Read the model definition and answer for the solid it produces. Units are mm, in the model's axes. Face numbers are marked on the shaded views. A direction names the side the tool comes from. Coordinates: 2 decimals unless noted, no trailing zeros. Loops run counter-clockwise (first coordinate to the right, second up) from the corner with the lowest first, then second, coordinate; pieces in that order, holes last.
Q1. Section C-C (y = 2.25) is taken. Give the vertices of the cut face in (x, z).
Q2. Flat-ended cylindrical pins translate along their axes: P1, Ø1.5, axis at y = 2.5, z = -3.5, coming from the +X side; P2, Ø3, axis at y = 8.5, z = 10, coming from the -X side; P3, Ø8, axis at x = -60.5, z = -10, coming from the -Y side. Find the tip coordinate at first contact, or state that the pin passes through.
Q3. Section D-D (z = -10.5) is taken. Give the vertices of the cut face in (x, y), then the cut area to 3 significant figures.
Q4. Section A-A (z = 0) is taken. Give the vertices of the cut face in (x, y), then the cut area to 3 significant figures.
Q5. Straight lines are drawn through the part: line 1 (Z direction, x = 5, y = 21.25); line 2 (X direction, y = 3.75, z = -0.25); line 3 (Z direction, x = 8, y = 21.75). For each, find the intervals that lie inside material, in ascending order.
Q6. Section B-B (y = 11.3) is taken. Give the vertices of the cut face in (x, z), then the cut area to 3 significant figures.
Q7. Which of the six approach directions +Z, -Z, +X, -X, +Y, -Y give full straight-line access (tool end or side, diameter ignored) to the marked faces 1 and 2?
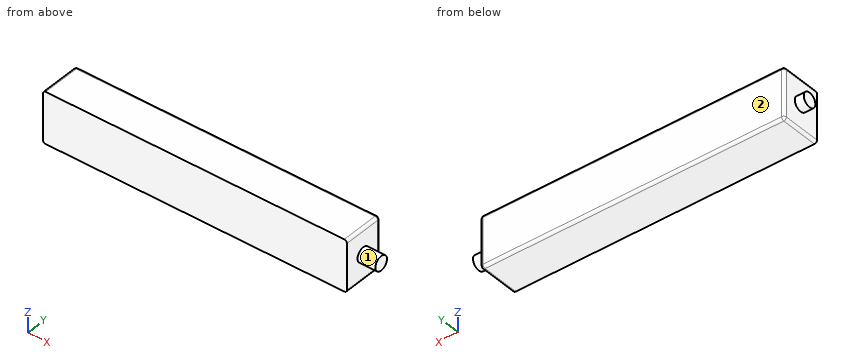
from build123d import *

# Parameters (mm, degrees)
SKETCH1_W           = 170
SKETCH1_H           = 28.6
BOSS_EXTRUDE1_DEPTH = 22.6
SKETCH2_R           = 4
BOSS_EXTRUDE2_DEPTH = 10
SKETCH3_R           = 4
BOSS_EXTRUDE3_DEPTH = 5
FILLET1_R           = 1.5


with BuildPart() as part:
    # Sketch1 → Boss-Extrude1 (new body)
    with BuildSketch(Plane(origin=(0, 0, 0), x_dir=(1, 0, 0), z_dir=(0, 1, 0))):
        Rectangle(SKETCH1_W, SKETCH1_H)
    extrude(amount=BOSS_EXTRUDE1_DEPTH)

    # Sketch2 → Boss-Extrude2 (add)
    with BuildSketch(Plane(origin=(85, 0, 0), x_dir=(0, 0, -1), z_dir=(1, 0, 0))):
        with Locations((0, 11.3)):
            Circle(SKETCH2_R)
    extrude(amount=BOSS_EXTRUDE2_DEPTH)

    # Sketch3 → Boss-Extrude3 (add)
    with BuildSketch(Plane.ZY.offset(85)):
        with Locations((0, 11.3)):
            Circle(SKETCH3_R)
    extrude(amount=BOSS_EXTRUDE3_DEPTH)

    # Fillet1
    fillet1_edges = [part.edges().sort_by_distance(p)[0] for p in [
        (85, 22.6, 0),
        (0, 22.6, -14.3),
        (-85, 22.6, 0),
        (0, 22.6, 14.3),
        (-85, 11.3, -14.3),
        (85, 11.3, -14.3),
        (85, 11.3, 14.3),
        (-85, 11.3, 14.3),
    ]]
    fillet(fillet1_edges, radius=FILLET1_R)


solid = part.part
Numbers:
1. outline: (-85, -12.8) arc R1.5 ccw to (-83.5, -14.3) - (83.5, -14.3) arc R1.5 ccw to (85, -12.8) - (85, 12.8) arc R1.5 ccw to (83.5, 14.3) - (-83.5, 14.3) arc R1.5 ccw to (-85, 12.8) - close
2. P1: stops at x = 85
2. P2: stops at x = -85
2. P3: stops at y = 0
3. outline: (-85, 0) - (85, 0) - (85, 21.1) arc R1.5 ccw to (83.5, 22.6) - (-83.5, 22.6) arc R1.5 ccw to (-85, 21.1) - close
3. area: 3,840 mm2
4. outline: (-90, 7.3) - (-85, 7.3) - (-85, 0) - (85, 0) - (85, 7.3) - (95, 7.3) - (95, 15.3) - (85, 15.3) - (85, 21.1) arc R1.5 ccw to (83.5, 22.6) - (-83.5, 22.6) arc R1.5 ccw to (-85, 21.1) - (-85, 15.3) - (-90, 15.3) - close
4. area: 3,960 mm2
5. line 1: z = -14.29 to 14.29
5. line 2: x = -85 to 85
5. line 3: z = -14.15 to 14.15
6. outline: (-90, -4) - (-85, -4) - (-85, -12.8) arc R1.5 ccw to (-83.5, -14.3) - (83.5, -14.3) arc R1.5 ccw to (85, -12.8) - (85, -4) - (95, -4) - (95, 4) - (85, 4) - (85, 12.8) arc R1.5 ccw to (83.5, 14.3) - (-83.5, 14.3) arc R1.5 ccw to (-85, 12.8) - (-85, 4) - (-90, 4) - close
6. area: 4,980 mm2
7. face 1: +X
7. face 2: +Z, -Z, +X, -X, +Y
